Solid Edge part; units mm, degrees
sketch "Sketch1" plane through (0, 0, 0) normal (1, 0, 0) x (0, 1, 0)
  circle A0 centre (0, 0) radius 11
  line L0 (10.238, -10.9628) -> (14.6087, 3.404)
  line L1 (14.6087, 3.404) -> (4.3353, 14.3598)
  line L2 (4.3353, 14.3598) -> (-10.2618, 10.9406)
  line L3 (-10.2618, 10.9406) -> (-14.6087, -3.404)
  line L4 (-14.6087, -3.404) -> (-4.3883, -14.3437)
  line L5 (-4.3883, -14.3437) -> (10.238, -10.9628)
extrude "Protrusion1" add sketch "Sketch1" against normal blind 16
cosmetic_thread "Thread1"
sketch "Sketch2" plane through (-16, 0, 0.0081) normal (-1, 0, 0) x (0, -0.9743092, -0.2252144)
  circle A0 centre (0.0018, -0.0078) radius 6.5
  circle A1 centre (0.0018, -0.0078) radius 11
extrude "ExtrudedProtrusion_2" add sketch "Sketch2" against normal blind 1
sketch "Sketch3" plane through (0, 0, 0) normal (1, 0, 0) x (0, 1, 0)
  circle A0 centre (0, 0) radius 3.5
  circle A1 centre (0, 0) radius 4.5
extrude "ExtrudedProtrusion_4" add sketch "Sketch3" against normal blind 110
sketch "Sketch4" plane through (-15, 0, 0) normal (1, 0, 0) x (0, 0, 1)
  circle A0 centre (0, 0) radius 8.7483
  circle A1 centre (0, 0) radius 4.5
extrude "ExtrudedProtrusion_5" add sketch "Sketch4" along normal blind 1
cosmetic_thread "Thread_3" thread depth 15
Design review of the part built by this model. Coordinates are the model's own, in mm. A direction names the side the tool comes from. Give positions to 0.01 mm unless a question says otherwise; leave off trailing zeros. Write each loop counter-clockwise with the first axis right and the second up, starting at its lowest first coordinate (ties: lowest second). Pieces come first, ordered by that corner, then holes. Notation, with made-up numbers: M 70,-35.75 L 102,-35.75 A26 cw 102,2.25 Z; hole C 24,39.5 d8. An arc over 180 degrees is marked long. Answer as a JSON object with one key per item and string values. Group by question number.
1) Mouldability with a two-part tool opening along Y and no side actions: class faces 4 (the face through (-6.9, -0.59, 4.46)), 5 (the face through (-7.89, 9.54, 8.81)), 6 (the face through (-7.888, -12.405, 3.869)), 7 (the face through (-110, 4, 0)) as released by +Y, released by -Y, zero draft, split by the parting line, or undercut.
2) For line 1 along Z through (x, y) = (-22.5, 0); line 2 along Z through (x, y) = (-4.5, 3); line 3 along X through (y, z) = (11, 3.5), list the stretches that pass through material, from the lowest coordinate up.
3) We need section B-B (z = 1.75). Give the boundary of the cut face in (x, y).
4) We need section C-C (x = -34). Give the boundary of the cut face in (y, z).
5) We need section A-A (y = 0). Give the boundary of the cut face in (x, z), and give its area (3 significant figures).
6) Tool access review of faces 1 (the face through (-15.5, -1.6, -6.3)), 2 (the face through (0, -11, 2)), 3 (the face through (-14, 4, 4)): name each direction out of +Z, -Z, +X, -X, +Y, -Y from which nothing blocks a thin tool from reaching the whole face with its end or side.
7) Clearance check with flat-ended pins moving along their axes: pin 1 Ø3 at (x, y) = (-30.5, 5) entering from -Z; pin 2 Ø1 at (y, z) = (-1, -7.5) entering from -X; pin 3 Ø1 at (x, y) = (-90, -5.5) entering from +Z; pin 4 Ø1.5 at (x, z) = (-50, 3.5) entering from +Y. State where each tip first meets the part, or that it passes through.
Answer key:
{
 "1": {"face 4": "undercut", "face 5": "released by +Y", "face 6": "released by -Y", "face 7": "zero draft"},
 "2": {"line 1": "z = -4.5 to -3.5, 3.5 to 4.5", "line 2": "z = -12.64 to -10.58, -3.35 to -1.8, 1.8 to 3.35, 10.58 to 14.05", "line 3": "x = -16 to 0"},
 "3": {"outline": "M -110,-4.15 L -15,-4.15 L -15,-6.26 L -16,-6.26 L -16,-13.05 L 0,-13.05 L 0,-10.86 L -15,-10.86 L -15,-8.57 L -14,-8.57 L -14,-4.15 L 0,-4.15 L 0,-3.03 L -110,-3.03 Z; M -110,3.03 L 0,3.03 L 0,4.15 L -14,4.15 L -14,8.57 L -15,8.57 L -15,10.86 L 0,10.86 L 0,14.11 L -16,14.11 L -16,6.26 L -15,6.26 L -15,4.15 L -110,4.15 Z"},
 "4": {"outline": "C 0,0 d9; hole C 0,0 d7"},
 "5": {"outline": "M -110,-4.5 L -15,-4.5 L -15,-6.5 L -16,-6.5 L -16,-13.33 L 0,-13.33 L 0,-11 L -15,-11 L -15,-8.75 L -14,-8.75 L -14,-4.5 L 0,-4.5 L 0,-3.5 L -110,-3.5 Z; M -110,3.5 L 0,3.5 L 0,4.5 L -14,4.5 L -14,8.75 L -15,8.75 L -15,11 L 0,11 L 0,13.34 L -16,13.34 L -16,6.5 L -15,6.5 L -15,4.5 L -110,4.5 Z", "area": "312 mm²"},
 "6": {"face 1": "-X", "face 2": "+Z, -Z, +X, +Y, -Y", "face 3": "+X"},
 "7": {"pin 1": "stops at z = -2.83", "pin 2": "stops at x = -16", "pin 3": "passes through", "pin 4": "stops at y = 3.56"}
}
